```python
from build123d import *

# Parameters (mm, degrees)
BOSS_EXTRUDE1_DEPTH          = 3.175
F_1_4_CLEARANCE_HOLE1_D      = 6.7564
F_10_0_1935_DIAMETER_HOLE1_D = 4.9149


with BuildPart() as part:
    # Sketch1 → Boss-Extrude1 (new body)
    with BuildSketch(Plane(origin=(0, 687.523670024, 112.992800714), x_dir=(1, 0, 0), z_dir=(0, 0.9867625124381891, 0.16217195826243377))):
        with BuildLine():
            Line((-76.2, -1167.779230682), (-76.2, -939.179230682))
            ThreePointArc((-76.2, -939.179230682), (-72.480256121, -930.198974561), (-63.5, -926.479230682))
            Line((-63.5, -926.479230682), (63.5, -926.479230682))
            ThreePointArc((63.5, -926.479230682), (72.480256121, -930.198974561), (76.2, -939.179230682))
            Line((76.2, -939.179230682), (76.2, -1167.779230682))
            ThreePointArc((76.2, -1167.779230682), (72.480256121, -1176.759486803), (63.5, -1180.479230682))
            Line((63.5, -1180.479230682), (-63.5, -1180.479230682))
            ThreePointArc((-63.5, -1180.479230682), (-72.480256121, -1176.759486803), (-76.2, -1167.779230682))
        make_face()
    extrude(amount=BOSS_EXTRUDE1_DEPTH)

    # 1/4 Clearance Hole1 (through all)
    with Locations(Plane(origin=(0, 690.656641001, 113.507696681), x_dir=(1, 0, 0), z_dir=(0, 0.9867625124381894, 0.16217195826243377))):
        with Locations((-63.5, -1167.779230682), (63.5, -1167.779230682), (63.5, -939.179230682), (-63.5, -939.179230682)):
            Hole(F_1_4_CLEARANCE_HOLE1_D / 2)

    # #10 (0.1935) Diameter Hole1 (through all)
    with Locations(Plane(origin=(0, 690.656641001, 113.507696681), x_dir=(1, 0, 0), z_dir=(0, 0.9867625124381891, 0.1621719582624338))):
        with Locations((38.1, -1142.379230682), (-38.1, -1142.379230682), (38.1, -1066.179230682), (-38.1, -1066.179230682)):
            Hole(F_10_0_1935_DIAMETER_HOLE1_D / 2)


solid = part.part
```
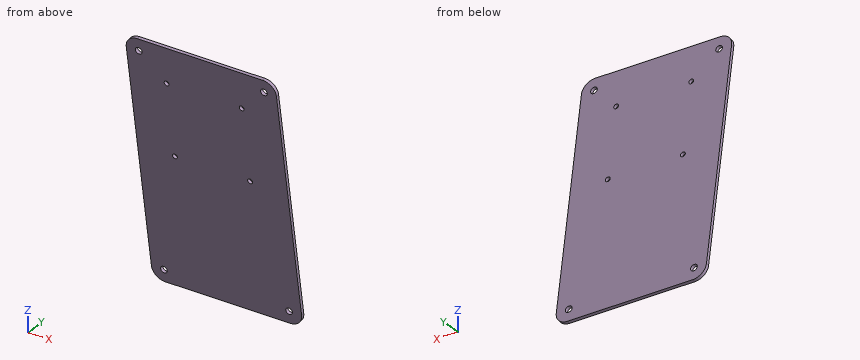
Build history of the part. All positions in model axes, mm. Give positions to 0.01 mm unless a question says otherwise; leave off trailing zeros. Loops run counter-clockwise (first coordinate to the right, second up) from the corner with the lowest first, then second, coordinate; pieces in that order, holes last.
1) Probe line 1 along Y through (x, z) = (57.5, 1230); line 2 along Y through (x, z) = (66, 1118). List the from-to ranges inside material, lowest first.
Values follow:
line 1: y = 503.95 to 507.16
line 2: y = 522.35 to 525.57
2) Drop flat-ended pins along their axis: P1, Ø3, axis at x = 32, z = 1079, coming from the -Y side; P2, Ø4, axis at x = 10, z = 1099.5, coming from the -Y side (3 decimals); P3, Ø1, axis at x = 47, z = 1065.5, coming from the +Y side. Give the stop position or say it passes through.
Values follow:
P1: stops at y = 528.52
P2: stops at y = 525.065
P3: stops at y = 534.28
3) Band-saw the part on B-B on z = 1156.5. List the corners of the cut face in (x, y).
Values follow:
outline: (-76.2, 516.03) - (76.2, 516.03) - (76.2, 519.24) - (-76.2, 519.24) - close
4) Band-saw the part on A-A on x = 50. List the corners of the cut face in (y, z).
Values follow:
outline: (496.08, 1277.85) - (537.27, 1027.21) - (540.41, 1027.72) - (499.22, 1278.36) - close
